from build123d import *

# Parameters (mm, degrees)
F0_W     = 65
F0_H     = 50
F1_DEPTH = 20
F2_R     = 12.5
F3_DEPTH = 10
F4_D     = 11
F4_DEPTH = 60
F4_TIP   = 3.3047334047
F6_D     = 6.8
F6_DEPTH = 23.75
F6_TIP   = 2.0429261047
F7_D     = 8
F7_DEPTH = 20
F7_TIP   = 2.4034424761


with BuildPart() as f1:
    # F0 (on Front) → F1 (new body, symmetric)
    with BuildSketch(Plane.XZ):
        Rectangle(F0_W, F0_H)
    extrude(amount=F1_DEPTH, both=True)

    # F2 (on face) → F3 (join)
    with BuildSketch(Plane.XZ.offset(20)):
        Circle(F2_R)
    extrude(amount=F3_DEPTH)

    # F4 (one way)
    with BuildSketch(Plane.XZ):
        with Locations((0, 0)):
            Circle(F4_D / 2)
    extrude(amount=-F4_DEPTH, mode=Mode.SUBTRACT)
    with Locations(Plane.XZ):
        with Locations((0, 0)):
            with Locations((0, 0, -(F4_DEPTH + F4_TIP / 2))):  # 118° drill point
                Cone(0, F4_D / 2, F4_TIP, mode=Mode.SUBTRACT)

    # F6
    with Locations(Plane(origin=(0, 20, 0), x_dir=(-1, 0, 0), z_dir=(0, 1, 0))):
        with Locations((-22.5, -17.5), (22.5, 17.5)):
            Hole(F6_D / 2, depth=F6_DEPTH)
            with Locations((0, 0, -(F6_DEPTH + F6_TIP / 2))):  # 118° drill point
                Cone(0, F6_D / 2, F6_TIP, mode=Mode.SUBTRACT)

    # F7
    with Locations(Plane(origin=(0, 20, 0), x_dir=(-1, 0, 0), z_dir=(0, 1, 0))):
        with Locations((-22.5, 17.5), (22.5, -17.5)):
            Hole(F7_D / 2, depth=F7_DEPTH)
            with Locations((0, 0, -(F7_DEPTH + F7_TIP / 2))):  # 118° drill point
                Cone(0, F7_D / 2, F7_TIP, mode=Mode.SUBTRACT)


solid = f1.part
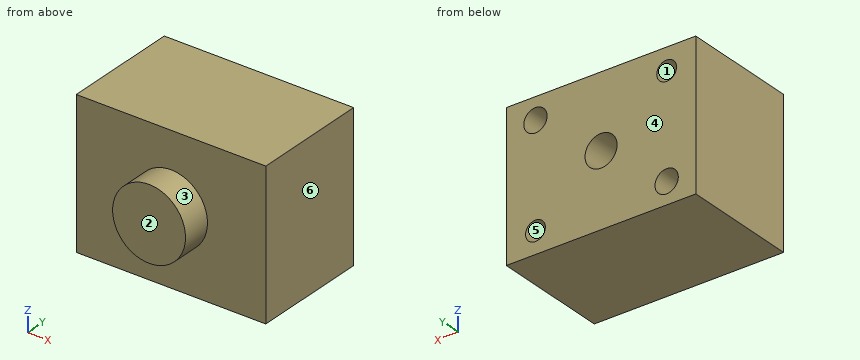
CAD build for the part. Positions are in the model's coordinates, mm. Face numbers are marked on the shaded views. A direction names the side the tool comes from. Coordinates: 2 decimals unless noted, no trailing zeros. Loops run counter-clockwise (first coordinate to the right, second up) from the corner with the lowest first, then second, coordinate; pieces in that order, holes last. Notation, with made-up numbers: (-27, 2) -> (-14, 2) arc R8 cw to (-14, 9) -> close; hole circle Ø10 at (56.5, -11). An arc over 180 degrees is marked (long way). One line per item, written item: value.
1. Slice it at C-C on x = -14.5. Write the cut outline in (y, z), and give its area (3 significant figures).
Answers:
outline: (-20, -25) -> (20, -25) -> (20, 25) -> (-20, 25) -> close
area: 2,000 mm^2
2. Slice it at A-A on y = 14.5. Write the cut outline in (x, z), and give its area (3 significant figures).
Answers:
outline: (-32.5, -25) -> (32.5, -25) -> (32.5, 25) -> (-32.5, 25) -> close; hole circle Ø8 at (-22.5, -17.5); hole circle Ø6.8 at (-22.5, 17.5); hole circle Ø11 at (0, 0); hole circle Ø8 at (22.5, 17.5); hole circle Ø6.8 at (22.5, -17.5)
area: 2,980 mm^2
3. Slice it at D-D on z = -10.5. Write the cut outline in (x, y).
Answers:
outline: (-32.5, -20) -> (-6.78, -20) -> (-6.78, -30) -> (6.78, -30) -> (6.78, -20) -> (32.5, -20) -> (32.5, 20) -> (-32.5, 20) -> close
4. Slice it at B-B on z = 0. Write the cut outline in (x, y).
Answers:
outline: (-32.5, -20) -> (-12.5, -20) -> (-12.5, -30) -> (12.5, -30) -> (12.5, -20) -> (32.5, -20) -> (32.5, 20) -> (5.5, 20) -> (5.5, 0) -> (-5.5, 0) -> (-5.5, 20) -> (-32.5, 20) -> close
5. Which spindle directions (+Z, -Z, +X, -X, +Y, -Y) get a long thin tool onto all of the face, cutting with end or side? Do the marked faces 1, 2 and 3. Say none if no direction does.
Answers:
face 1: +Y
face 2: +Z, -Z, +X, -X, -Y
face 3: -Y
6. Flat gauge pin, fed straight in: P1, Ø5, axis at x = 22.5, z = 17.5, coming from the -Y side. Where does the tip first touch, or does it go through?
Answers:
P1: stops at y = -20
7. Pull direction X, two halves, no side cores. Call the marked faces 4, 5 and 6: pulls with the +X half, pulls with the -X half, needs draft (parallel to the pull), parting line crosses it, or undercut.
Answers:
face 4: needs draft
face 5: undercut
face 6: pulls with the +X half
8. Drill centre lines: line 1 (X direction, y = 1.5, z = 17.5); line 2 (Z direction, x = 22.5, y = 6.75); line 3 (X direction, y = 8.5, z = -17.5). Where is each one in solid material? Low to high. Write a range as [from, to].
Answers:
line 1: x = [-32.5, -25.9], [-19.1, 18.5], [26.5, 32.5]
line 2: z = [-25, -20.9], [-14.1, 13.5], [21.5, 25]
line 3: x = [-32.5, -26.5], [-18.5, 19.1], [25.9, 32.5]
